```python
from build123d import *

# Parameters (mm, degrees)
SKETCH_1_R          = 6
EXTRUDE_1_DEPTH     = 15
EXTRUDE_2_DEPTH     = 2
SKETCH_3_R          = 7
EXTRUDE_3_DEPTH     = 1
CHAMFER_1_SIZE      = 1
FILLET_1_R          = 1
SKETCH_4_R          = 5
CUT_EXTRUDE_1_DEPTH = 10


with BuildPart() as part:
    # 草图1 → 凸台-拉伸1 (new body)
    with BuildSketch(Plane.XY):
        Circle(SKETCH_1_R)
    extrude(amount=EXTRUDE_1_DEPTH)

    # 草图2 → 凸台-拉伸2 (add)
    with BuildSketch(Plane.XY.offset(15)):
        Polygon((4.70381444, 7.950312136), (-4.533265058, 8.048778867), (-9.237079497, 0.098466732), (-4.70381444, -7.950312136), (4.533265058, -8.048778867), (9.237079497, -0.098466732), align=None)
    extrude(amount=EXTRUDE_2_DEPTH)

    # 草图3 → 凸台-拉伸3 (add)
    with BuildSketch(Plane.XY.offset(17)):
        Circle(SKETCH_3_R)
    extrude(amount=EXTRUDE_3_DEPTH)

    # 倒角1
    chamfer_1_edges = [part.edges().sort_by_distance(p)[0] for p in [
        (-6, 0, 0),
        (-7, 0, 18),
        (6.970446968, 3.925922702, 17),
        (0.085274691, 7.999545501, 17),
        (-6.885172277, 4.073622799, 17),
        (-6.970446968, -3.925922702, 17),
        (-0.085274691, -7.999545501, 17),
        (6.885172277, -4.073622799, 17),
    ]]
    chamfer(chamfer_1_edges, length=CHAMFER_1_SIZE - 0.0001)  # a hair under: the kernel refuses the full size

    # 圆角1
    fillet_1_edges = [part.edges().sort_by_distance(p)[0] for p in [
        (-6.885172277, 4.073622799, 16.0001),
        (0.085274691, 7.999545501, 16.0001),
        (6.970446968, 3.925922702, 16.0001),
        (6.885172277, -4.073622799, 16.0001),
        (-6.970446968, -3.925922702, 16.0001),
        (-0.085274691, -7.999545501, 16.0001),
    ]]
    fillet(fillet_1_edges, radius=FILLET_1_R)

    # 草图4 → 切除-拉伸1 (cut)
    with BuildSketch(Plane(origin=(0, 0, 0), x_dir=(-1, 0, 0), z_dir=(0, 0, -1))):
        Circle(SKETCH_4_R)
    extrude(amount=-CUT_EXTRUDE_1_DEPTH, mode=Mode.SUBTRACT)


solid = part.part
```
Work out the finished part from the listing and answer in its coordinate system (mm). A direction names the side the tool comes from. Coordinates: 2 decimals unless noted, no trailing zeros. Loops run counter-clockwise (first coordinate to the right, second up) from the corner with the lowest first, then second, coordinate; pieces in that order, holes last.
1) Flat-ended cylindrical pins translate along their axes: pin 1 (4 mm diameter, centred on x = -5, z = 12.5, fed in from +Y); pin 2 (1 mm diameter, centred on y = -1.5, z = 14, fed in from +X); pin 3 (1.5 mm diameter, centred on x = -7, z = 13.5, fed in from +Y); pin 4 (5 mm diameter, centred on x = -2.5, z = 5.5, fed in from -Y). Find the tip coordinate at first contact, or state that the pin passes through.
Results:
pin 1: stops at y = 5.2
pin 2: stops at x = 5.92
pin 3: passes through
pin 4: stops at y = -6
2) Section A-A (z = 15.25) is taken. Give the vertices of the cut face in (x, y).
Results:
outline: (-9.24, 0.1) - (-4.7, -7.95) - (4.53, -8.05) - (9.24, -0.1) - (4.7, 7.95) - (-4.53, 8.05) - close
3) Consider probe 1 along Y at (x, z) = (0, 3.25); probe 2 along X at (y, z) = (3.75, 2.25); probe 3 along Z at (x, y) = (4.75, 5.5). Determine where each line is inside the solid, lowest interval first.
Results:
probe 1: y = -6 to -5, 5 to 6
probe 2: x = -4.68 to -3.31, 3.31 to 4.68
probe 3: z = 15 to 17
4) Section C-C (z = 10.5) is taken. Give the vertices of the cut face in (x, y), plus the area to 3 significant figures.
Results:
outline: circle Ø12 at (0, 0)
area: 113 mm2
5) Section B-B (z = 6.5) is taken. Give the vertices of the cut face in (x, y), plus the area to 3 significant figures.
Results:
outline: circle Ø12 at (0, 0); hole circle Ø10 at (0, 0)
area: 34.6 mm2
6) For faces 4 (the flat face through (6.301, -3.801, 16.642)), 5 (the flat face through (0, 0, 10)), determine the directions among +Z, -Z, +X, -X, +Y, -Y from which every point of the face is accessible in a straight line to the end or side of a thin tool.
Results:
face 4: +Z, +X, -Y
face 5: -Z
7) For a pull along X with two mould halves and no side action, classify faces 1 (the cylindrical face through (1.08, -4.88, 4.93)), 2 (the flat face through (7.15, 0.03, 17)), 3 (the flat face through (6.85, -4.13, 15.29)) as +X half, -X half, draft (parallel to the pull), parting line (faces both ways), or undercut.
Results:
face 1: undercut
face 2: draft
face 3: +X half
